Geometry: final body of the model. Coordinates: model frame, mm. Face numbers are marked on the shaded views. A direction names the side the tool comes from. Give positions to 0.01 mm unless a question says otherwise; leave off trailing zeros. Order: outer loops, then holes, each group sorted by start corner. A loop starts at its lowest first (then second) coordinate and runs counter-clockwise, first axis right, second up. Notation, with made-up numbers: (76.25, 39) - (101.25, 39) arc R13 cw to (101.25, 43) - close; hole circle Ø11 at (48.5, -12.5). An arc over 180 degrees is marked (long way). Write item = value, one per line. Start each with the question number.
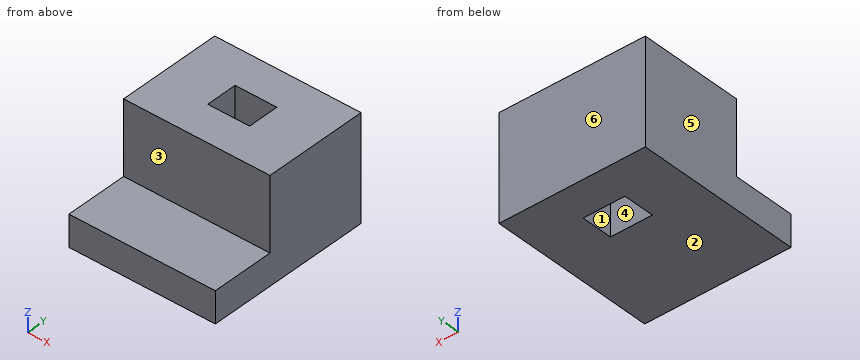
from build123d import *

# Parameters (mm, degrees)
F0_W     = 14
F0_H     = 16
F1_DEPTH = 10
F2_W     = 14
F2_H     = 6
F3_DEPTH = 7
F4_W     = 4
F4_H     = 3
F5_DEPTH = 10.001


with BuildPart() as f1:
    # F0 (on Top) → F1 (new body)
    with BuildSketch(Plane.XY):
        with Locations((7, -8)):
            Rectangle(F0_W, F0_H)
    extrude(amount=F1_DEPTH)

    # F2 (on face) → F3 (cut)
    with BuildSketch(Plane.XY.offset(10)):
        with Locations((7, -13)):
            Rectangle(F2_W, F2_H)
    extrude(amount=-F3_DEPTH, mode=Mode.SUBTRACT)

    # F4 (on face) → F5 (cut, through all)
    with BuildSketch(Plane.XY.offset(10)):
        with Locations((7, -5)):
            Rectangle(F4_W, F4_H)
    extrude(amount=-F5_DEPTH, mode=Mode.SUBTRACT)


solid = f1.part
Q1. Section A-A, the plane x = 6.25. Return the cut outline in (y, z).
Q2. Section B-B, the plane y = -6. Return the cut outline in (x, z).
Q3. Section D-D, the plane x = 12. Return the cut outline in (y, z), then the cut area to 3 significant figures.
Q4. Material intervals for line 1 along X through (y, z) = (-5.75, 8); line 2 along Y through (x, z) = (8.75, 8.5); line 3 along Y through (x, z) = (8.25, 2.75), sorted ascending. Write a range as from..to.
Q5. Section C-C, the plane z = 3.75. Return the cut outline in (x, y), then the cut area to 3 significant figures.
Q6. Set-up query: the marked faces 1, 2 and 3. Return all of +Z, -Z, +X, -X, +Y, -Y with unobstructed straight access to the full face (end or side cutting, diameter ignored); none if empty.
Q7. Pull-direction query (X, two-part tool) for the marked faces 4, 5 and 6; classes: +X half, -X half, draft (parallel to the pull), parting line (faces both ways), or undercut.
Q8. Contact query for flat-ended pins moving along their axis: pin 1 (1.8 mm diameter, centred on x = 7.5, y = -13, fed in from +Z); pin 2 (1.2 mm diameter, centred on x = 7, z = 6, fed in from -Y). Output: stop coordinate, or through.
The answers:
q1.outline = (-16, 0) - (-6.5, 0) - (-6.5, 10) - (-10, 10) - (-10, 3) - (-16, 3) - close; (-3.5, 0) - (0, 0) - (0, 10) - (-3.5, 10) - close
q2.outline = (0, 0) - (5, 0) - (5, 10) - (0, 10) - close; (9, 0) - (14, 0) - (14, 10) - (9, 10) - close
q3.outline = (-16, 0) - (0, 0) - (0, 10) - (-10, 10) - (-10, 3) - (-16, 3) - close
q3.area = 118 mm²
q4.line_1 = 0..5, 9..14
q4.line_2 = -10..-6.5, -3.5..0
q4.line_3 = -16..-6.5, -3.5..0
q5.outline = (0, -10) - (14, -10) - (14, 0) - (0, 0) - close; hole (5, -6.5) - (9, -6.5) - (9, -3.5) - (5, -3.5) - close
q5.area = 128 mm²
q6.face_1 = +Z, -Z
q6.face_2 = -Z, +X, -X, +Y, -Y
q6.face_3 = +Z, +X, -X, -Y
q7.face_4 = undercut
q7.face_5 = -X half
q7.face_6 = draft
q8.pin_1 = 3
q8.pin_2 = -10
